Could you check a few things on this model? Use its own coordinates, in mm. Face numbers are marked on the shaded views. A direction names the side the tool comes from. Give positions to 0.01 mm unless a question says otherwise; leave off trailing zeros. Write each loop counter-clockwise with the first axis right and the second up, starting at its lowest first coordinate (ties: lowest second). Pieces come first, ordered by that corner, then holes. Notation, with made-up numbers: M 82,68.5 L 100,68.5 A8 ccw 100,78.5 Z; hole C 27.25,23 d1. An arc over 180 degrees is marked long. One line per item, written item: value.
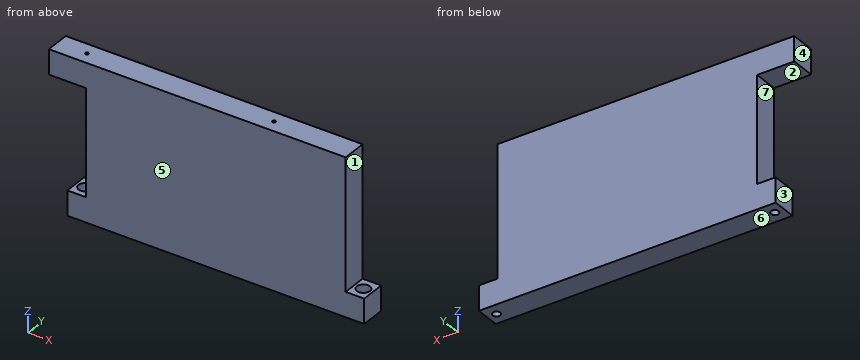
```python
from build123d import *

# Parameters (mm, degrees)
F0_W      = 304.8
F0_H      = 25.4
F1_DEPTH  = 160.02
F2_W      = 19.05
F2_H      = 25.4
F3_DEPTH  = 134.62
F4_R      = 3.970807
F4_R_2    = 4.064
F5_DEPTH  = 25.401
F4_R_3    = 6.731
F6_DEPTH  = 12.7
F7_W      = 25.4
F7_H      = 25.4
F8_DEPTH  = 38.1
F9_R      = 1.7272
F10_DEPTH = 19.05


with BuildPart() as f1:
    # F0 (on Top) → F1 (new body)
    with BuildSketch(Plane.XY):
        Rectangle(F0_W, F0_H)
    extrude(amount=F1_DEPTH)

    # F2 (on face) → F3 (cut)
    with BuildSketch(Plane.XY.offset(160.02)):
        with Locations((-142.875, 0)):
            Rectangle(F2_W, F2_H)
        with Locations((142.875, 0)):
            Rectangle(F2_W, F2_H)
    extrude(amount=-F3_DEPTH, mode=Mode.SUBTRACT)

    # F4 (on face) → F5 (cut, through all)
    with BuildSketch(Plane.XY.offset(25.4)):
        with Locations((142.875, 0)):
            Circle(F4_R)
        with Locations((-142.875, 0)):
            Circle(F4_R_2)
    extrude(amount=-F5_DEPTH, mode=Mode.SUBTRACT)

    # F4 (on face) → F6 (cut)
    with BuildSketch(Plane.XY.offset(25.4)):
        with Locations((-142.875, 0)):
            Circle(F4_R_3)
        with Locations((-142.875, 0)):
            Circle(F4_R_2, mode=Mode.SUBTRACT)
        with Locations((142.875, 0)):
            Circle(F4_R_3)
        with Locations((142.875, 0)):
            Circle(F4_R, mode=Mode.SUBTRACT)
    extrude(amount=-F6_DEPTH, mode=Mode.SUBTRACT)

    # F7 (on face) → F8 (join)
    with BuildSketch(Plane(origin=(-133.35, 0, 0), x_dir=(0, -1, 0), z_dir=(-1, 0, 0))):
        with Locations((0, 147.32)):
            Rectangle(F7_W, F7_H)
    extrude(amount=F8_DEPTH)

    # F9 (on face) → F10 (cut)
    with BuildSketch(Plane.XY.offset(160.02)):
        with Locations((-140.95, 0)):
            Circle(F9_R)
        with Locations((51.05, 0)):
            Circle(F9_R)
    extrude(amount=-F10_DEPTH, mode=Mode.SUBTRACT)


solid = f1.part
```
1) On a 3-axis mill with a long thin cutter (end or side, diameter ignored), from which of +Z, -Z, +X, -X, +Y, -Y can I reach the whole of each face in a straight line? I mean the marked faces 1, 2, 3 and 4. Say none if no direction works.
Outcome:
face 1: +Z, +X, +Y, -Y
face 2: -X, +Y, -Y
face 3: -Z, -X, +Y, -Y
face 4: +Z, -Z, -X, +Y, -Y
2) We'd pull the mould along Z, two halves only. Please class the marked faces 5, 6 and 7: pulls with the +Z half, pulls with the -Z half, needs draft (parallel to the pull), parting line crosses it, or undercut.
Outcome:
face 5: needs draft
face 6: pulls with the -Z half
face 7: undercut
3) I'm going to push flat-ended pins straight in: pin 1 (10 mm diameter, centred on x = -54.5, y = 3, fed in from -Z); pin 2 (4 mm diameter, centred on x = 141, y = -3, fed in from +Z); pin 3 (6.5 mm diameter, centred on x = -142.875, y = 0, fed in from -Z); pin 4 (1 mm diameter, centred on x = 51, y = 0.5, fed in from +Z). Where does each tip first touch, or does it pass through?
Outcome:
pin 1: stops at z = 0
pin 2: stops at z = 12.7
pin 3: stops at z = 134.62
pin 4: stops at z = 140.97
4) If we section it at A-A, the plane z = 87: Write out the boundary of the cut face in (x, y), then the cut area to 3 significant figures.
Outcome:
outline: M -133.35,-12.7 L 133.35,-12.7 L 133.35,12.7 L -133.35,12.7 Z
area: 6,770 mm^2
5) Please list where these lines run through material, in increasing order: L1, parallel to Y at x = -140.95, z = 153; L2, parallel to Z at x = -144.5, y = -11.5; L3, parallel to X at y = -11, z = 21.5. Write a range as from..to.
Outcome:
L1: y = -12.7..-1.73, 1.73..12.7
L2: z = 0..25.4, 134.62..160.02
L3: x = -152.4..152.4
